Read the model definition and answer for the solid it produces. Units are mm, in the model's axes. Face numbers are marked on the shaded views. Coordinates: 2 decimals unless noted, no trailing zeros. Order: outer loops, then holes, each group sorted by start corner. A loop starts at its lowest first (then second) coordinate and runs counter-clockwise, first axis right, second up. Notation, with made-up numbers: M 26.25,-36 L 30.25,-36 A13 ccw 30.25,-20 Z; hole C 88,36.25 d4. An arc over 180 degrees is marked long. Write each question's results on one line, items separated by ' | '.
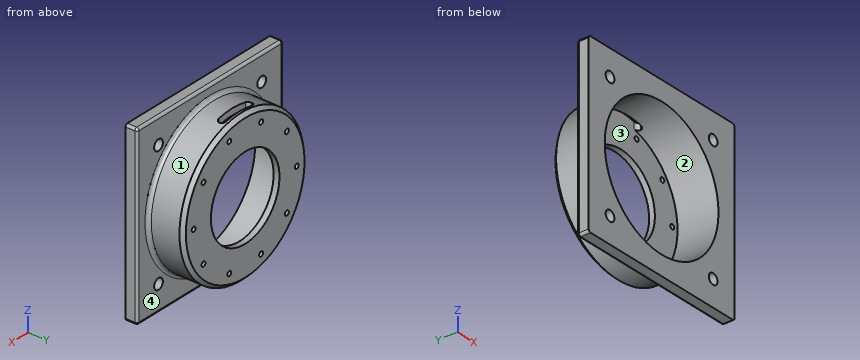
```python
from build123d import *

# Parameters (mm, degrees)
SKETCH_1_W          = 150
SKETCH_1_H          = 150
SKETCH_1_R          = 4.5
EXTRUDE_1_DEPTH     = 10
FILLET_1_R          = 2
FILLET_2_R          = 2
SKETCH_4_R          = 64
EXTRUDE_4_DEPTH     = 30
FILLET_5_R          = 3
SKETCH_11_R         = 35.25
CUT_EXTRUDE_2_DEPTH = 41
SKETCH_10_R         = 58.5
CUT_EXTRUDE_3_DEPTH = 35
SKETCH_12_R         = 2
CUT_EXTRUDE_4_DEPTH = 41
CHAMFER_2_SIZE      = 3
SKETCH_14_W         = 33.25
SKETCH_14_H         = 6.25
CUT_EXTRUDE_5_DEPTH = 9
FILLET_7_R          = 3


with BuildPart() as part:
    # Эскиз1 → Бобышка-Вытянуть1 (new body)
    with BuildSketch(Plane(origin=(0, 0, 0), x_dir=(1, 0, 0), z_dir=(0, 1, 0))):
        Rectangle(SKETCH_1_W, SKETCH_1_H)
        with Locations((53.033008589, 53.033008589)):
            Circle(SKETCH_1_R, mode=Mode.SUBTRACT)
        with Locations((53.033008589, -53.033008589)):
            Circle(SKETCH_1_R, mode=Mode.SUBTRACT)
        with Locations((-53.033008589, -53.033008589)):
            Circle(SKETCH_1_R, mode=Mode.SUBTRACT)
        with Locations((-53.033008589, 53.033008589)):
            Circle(SKETCH_1_R, mode=Mode.SUBTRACT)
    extrude(amount=EXTRUDE_1_DEPTH)

    # Скругление1
    fillet_1_edges = [part.edges().sort_by_distance(p)[0] for p in [
        (-75, 5, -75),
        (75, 5, -75),
        (75, 5, 75),
        (-75, 5, 75),
    ]]
    fillet(fillet_1_edges, radius=FILLET_1_R)

    # Скругление2
    fillet_2_edges = [part.edges().sort_by_distance(p)[0] for p in [
        (-75, 10, 0),
        (0, 10, -75),
        (0, 10, 75),
        (75, 10, 0),
        (74.414213562, 10, 74.414213562),
        (-74.414213562, 10, 74.414213562),
        (74.414213562, 10, -74.414213562),
        (-74.414213562, 10, -74.414213562),
    ]]
    fillet(fillet_2_edges, radius=FILLET_2_R)

    # Эскиз4 → Бобышка-Вытянуть4 (add)
    with BuildSketch(Plane(origin=(0, 10, 0), x_dir=(1, 0, 0), z_dir=(0, 1, 0))):
        Circle(SKETCH_4_R)
    extrude(amount=EXTRUDE_4_DEPTH)

    # Скругление5
    fillet_5_edges = [part.edges().sort_by_distance(p)[0] for p in [
        (-64, 10, 0),
    ]]
    fillet(fillet_5_edges, radius=FILLET_5_R)

    # Эскиз11 → Вырез-Вытянуть2 (cut, through all)
    with BuildSketch(Plane(origin=(0, 40, 0), x_dir=(1, 0, 0), z_dir=(0, 1, 0))):
        Circle(SKETCH_11_R)
    extrude(amount=-CUT_EXTRUDE_2_DEPTH, mode=Mode.SUBTRACT)

    # Эскиз10 → Вырез-Вытянуть3 (cut)
    with BuildSketch(Plane.XZ):
        Circle(SKETCH_10_R)
    extrude(amount=-CUT_EXTRUDE_3_DEPTH, mode=Mode.SUBTRACT)

    # Эскиз12 → Вырез-Вытянуть4 (cut, through all)
    with BuildSketch(Plane(origin=(0, 40, 0), x_dir=(1, 0, 0), z_dir=(0, 1, 0))):
        with Locations((-53, 0)):
            Circle(SKETCH_12_R)
        with Locations((-42.877900702, 31.152618372)):
            Circle(SKETCH_12_R)
        with Locations((-16.377900702, 50.405995364)):
            Circle(SKETCH_12_R)
        with Locations((16.377900702, 50.405995364)):
            Circle(SKETCH_12_R)
        with Locations((42.877900702, 31.152618372)):
            Circle(SKETCH_12_R)
        with Locations((53, 0)):
            Circle(SKETCH_12_R)
        with Locations((42.877900702, -31.152618372)):
            Circle(SKETCH_12_R)
        with Locations((16.377900702, -50.405995364)):
            Circle(SKETCH_12_R)
        with Locations((-16.377900702, -50.405995364)):
            Circle(SKETCH_12_R)
        with Locations((-42.877900702, -31.152618372)):
            Circle(SKETCH_12_R)
    extrude(amount=-CUT_EXTRUDE_4_DEPTH, mode=Mode.SUBTRACT)

    # Фаска2
    chamfer_2_edges = [part.edges().sort_by_distance(p)[0] for p in [
        (-64, 40, 0),
    ]]
    chamfer(chamfer_2_edges, length=CHAMFER_2_SIZE)

    # Эскиз14 → Вырез-Вытянуть5 (cut)
    with BuildSketch(Plane.XY.offset(64)):
        with Locations((0, 31.875)):
            Rectangle(SKETCH_14_W, SKETCH_14_H)
    extrude(amount=-CUT_EXTRUDE_5_DEPTH, mode=Mode.SUBTRACT)

    # Скругление7
    fillet_7_edges = [part.edges().sort_by_distance(p)[0] for p in [
        (-16.625, 28.75, 58.945474725),
        (-16.625, 35, 58.945474725),
        (16.625, 35, 58.945474725),
        (16.625, 28.75, 58.945474725),
    ]]
    fillet(fillet_7_edges, radius=FILLET_7_R)


solid = part.part
```
(1) The part is cut by section C-C, the plane y = 19.5. Write down the section's boundary in (x, z).
Conclusion:
outline: C 0,0 d128; hole C 0,0 d117
(2) The part is cut by section A-A, the plane x = 0. Write down the section's boundary in (y, z), then the cut area to 3 significant figures.
Conclusion:
outline: M 0,-75 L 8,-75 A2 ccw 10,-73 L 10,-67 A3 cw 13,-64 L 37,-64 L 40,-61 L 40,-35.25 L 35,-35.25 L 35,-58.5 L 0,-58.5 Z; M 0,58.5 L 28.75,58.5 L 28.75,64 L 13,64 A3 cw 10,67 L 10,73 A2 ccw 8,75 L 0,75 Z; M 35,35.25 L 40,35.25 L 40,61 L 37,64 L 35,64 Z | area: 851 mm²
(3) The part is cut by section B-B, the plane z = 0. Count the separate pieces of the cut face and the enclosed holes in it, then the cut area to 3 significant figures.
Conclusion:
separate pieces: 4 | enclosed holes: 0 | area: 846 mm²
(4) Straight lines are drawn through the part: line 1 (X direction, y = 37.5, z = 0); line 2 (X direction, y = 37.5, z = -50); line 3 (Y direction, x = -39.5, z = 25). For each, find the intervals that lie inside material, in ascending order.
Conclusion:
line 1: -63.5 to -55, -51 to -35.25, 35.25 to 51, 55 to 63.5 | line 2: -39.14 to -18.34, -14.42 to 14.42, 18.34 to 39.14 | line 3: 35 to 40
(5) The mould has two halves that part along X. Classify the marked faces 1, 2, 3 and 4: pulls with the +X half, pulls with the -X half, needs draft (parallel to the pull), parting line crosses it, or undercut.
Conclusion:
face 1: parting line crosses it | face 2: undercut | face 3: undercut | face 4: needs draft
(6) Given pin 1 (2 mm diameter, centred on x = 57.5, y = 28.5, fed in from +Z); pin 2 (5 mm diameter, centred on x = -53, y = 20, fed in from +Z); pin 3 (10 mm diameter, centred on x = -40, y = 22.5, fed in from -Z), each flat-ended and moving along its own axis, determine where each tip first touches the part or whether it passes through.
Conclusion:
pin 1: z = 30.06 | pin 2: z = 39.32 | pin 3: z = -53.58
